Input: dimensioned drawing with shaded views. Units: mm. Origin: part minimum x, y, z. A direction names the side the tool comes from. Coordinates: 2 decimals unless noted, no trailing zeros. Loops run counter-clockwise (first coordinate to the right, second up) from the corner with the lowest first, then second, coordinate; pieces in that order, holes last.
Item 1: Section query C-C, the plane z = 4. Return the cut outline in (x, y).
Item 2: Pull-direction query (Z, two-part tool) for the marked faces 1, 2 and 3; classes: +Z half, -Z half, draft (parallel to the pull), parting line (faces both ways), or undercut.
Item 3: Section query B-B, the plane x = 5.5. Return the cut outline in (y, z).
Item 4: Reachability of the marked faces 4, 5 and 6 from +Z, -Z, +X, -X, +Y, -Y: full face, straight path, thin tool, end or side. Return the list, or none.
Item 5: Pin query (flat end, axial travel): pin 1 Ø3 at (x, y) = (11, 8) entering from -Z; pin 2 Ø1 at (x, z) = (27.5, 3.5) entering from -Y; pin 3 Ø6.5 at (x, y) = (28.5, 3) entering from -Z; pin 4 Ø2.5 at (x, z) = (5.5, 4) entering from -Y. Return the tip coordinate at first contact, or that it passes through.
Item 6: Section query D-D, the plane y = 7. Return the cut outline in (x, z).
Item 7: Line query: probe 1 along Z at (x, y) = (5.5, 10.5); probe 2 along X at (y, z) = (9.5, 6.75); probe 3 along Y at (x, z) = (5.5, 2). Output: solid intervals per line, ascending.
Item 8: Section query A-A, the plane y = 4.5. Return the cut outline in (x, z).
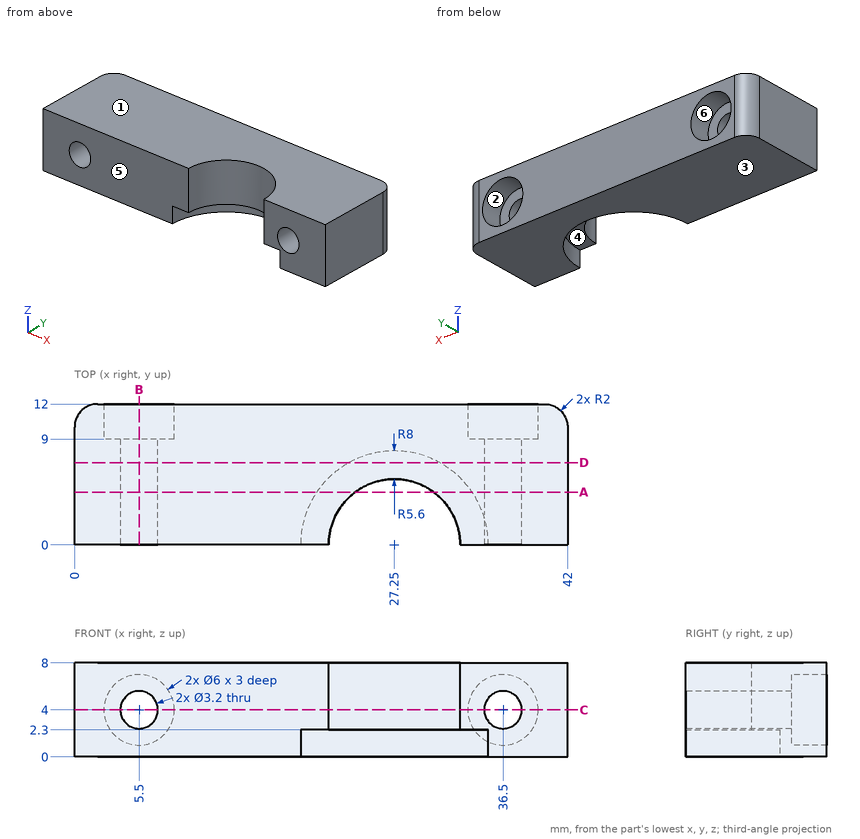
Verdict:
1. outline: (0, 0) - (3.9, 0) - (3.9, 9) - (2.5, 9) - (2.5, 12) - (2, 12) arc R2 ccw to (0, 10) - close; (7.1, 0) - (21.65, 0) arc R5.6 cw to (32.85, 0) - (34.9, 0) - (34.9, 9) - (33.5, 9) - (33.5, 12) - (8.5, 12) - (8.5, 9) - (7.1, 9) - close; (38.1, 0) - (42, 0) - (42, 10) arc R2 ccw to (40, 12) - (39.5, 12) - (39.5, 9) - (38.1, 9) - close
2. face 1: +Z half
2. face 2: undercut
2. face 3: -Z half
3. outline: (0, 0) - (12, 0) - (12, 1) - (9, 1) - (9, 2.4) - (0, 2.4) - close; (0, 5.6) - (9, 5.6) - (9, 7) - (12, 7) - (12, 8) - (0, 8) - close
4. face 4: -Z, -Y
4. face 5: +Z, -Z, +X, -X, -Y
4. face 6: +Y
5. pin 1: stops at z = 0
5. pin 2: stops at y = 5.55
5. pin 3: stops at z = 2.3
5. pin 4: passes through
6. outline: (0, 0) - (23.38, 0) - (23.38, 2.3) - (31.12, 2.3) - (31.12, 0) - (42, 0) - (42, 8) - (0, 8) - close; hole circle Ø3.2 at (5.5, 4); hole circle Ø3.2 at (36.5, 4)
7. probe 1: z = 0 to 1, 7 to 8
7. probe 2: x = 0 to 4.3, 6.7 to 35.3, 37.7 to 42
7. probe 3: y = 0 to 9
8. outline: (0, 0) - (20.64, 0) - (20.64, 2.3) - (23.92, 2.3) - (23.92, 8) - (0, 8) - close; (30.58, 2.3) - (33.86, 2.3) - (33.86, 0) - (42, 0) - (42, 8) - (30.58, 8) - close; hole circle Ø3.2 at (5.5, 4); hole circle Ø3.2 at (36.5, 4)
